Geometry check sheet. Reference: the model listing, model coordinates, mm. A direction names the side the tool comes from. Give positions to 0.01 mm unless a question says otherwise; leave off trailing zeros. Loops run counter-clockwise (first coordinate to the right, second up) from the corner with the lowest first, then second, coordinate; pieces in that order, holes last. Notation, with made-up numbers: (65, 75.5) -> (115, 75.5) arc R15 cw to (115, 79.5) -> close; hole circle Ø1 at (60.25, -26). An arc over 180 degrees is marked (long way). Write each question's results on one line, items separated by ' | '. Start each with the question number.
1) Draft check along X on faces 4 (the face through (67, 6, -75.8)), 5 (the face through (75.57, 6.08, -89.3)), 6 (the face through (56.019, 11.014, -79.626)), 7 (the face through (47, 10, -68)). Enter one of: pulls with the +X half, pulls with the -X half, needs draft (parallel to the pull), parting line crosses it, or undercut.
2) Sectioned sample at A-A on y = 1.5. Record the cut outline in (x, z), then the cut area to 3 significant figures.
3) Set-up check for faces 1 (the face through (62, 6, -61)), 2 (the face through (60, 5, -68)), 3 (the face through (37.92, 11.01, -78.84)): record each of +Z, -Z, +X, -X, +Y, -Y from which the full face is reachable in a straight line by a thin tool's end or side.
4) Depth check by flat-ended pin: pin 1 (13.5 mm diameter, centred on x = 43, z = -78.5, fed in from -Y); pin 2 (6 mm diameter, centred on y = 5.5, z = -60.5, fed in from +X); pin 3 (3 mm diameter, centred on x = 67, y = 8, fed in from +Z). Enter the tip coordinate at first touch or a pass-through.
5) Sectioned sample at C-C on z = -58.1. Record the cut outline in (x, y).
6) Scan lines: line 1 (X direction, y = 11.25, z = -58.1); line 2 (Z direction, x = 36.5, y = 11); line 3 (X direction, y = 3, z = -86). Record each from-to range of solid material in increasing order. Write a range as from..to.
7) Sectioned sample at B-B on x = 56.5. Record the cut outline in (y, z), then the cut area to 3 significant figures.
8) Sectioned sample at D-D on z = -81.5. Record the cut outline in (x, y).
```python
from build123d import *

# Parameters (mm, degrees)
SKETCH1_W           = 31
SKETCH1_H           = 45.4
BOSS_EXTRUDE1_DEPTH = 12
SKETCH2_W           = 27
SKETCH2_H           = 10
CUT_EXTRUDE1_DEPTH  = 57.268641356
SKETCH3_R           = 1.6
CUT_EXTRUDE2_DEPTH  = 10
SKETCH4_W           = 15
SKETCH4_H           = 12
BOSS_EXTRUDE2_DEPTH = 15
SKETCH5_R           = 1.6
CUT_EXTRUDE3_DEPTH  = 20
FILLET1_R           = 5


with BuildPart() as part:
    # Sketch1 → Boss-Extrude1 (new body)
    with BuildSketch(Plane(origin=(0, 0, 0), x_dir=(1, 0, 0), z_dir=(0, 1, 0))):
        with Locations((15.5, 22.7)):
            Rectangle(SKETCH1_W, SKETCH1_H)
    extrude(amount=BOSS_EXTRUDE1_DEPTH)

    # Sketch2 → Cut-Extrude1 (cut, through all)
    with BuildSketch(Plane.XY):
        with Locations((15.5, 5)):
            Rectangle(SKETCH2_W, SKETCH2_H)
    extrude(amount=-CUT_EXTRUDE1_DEPTH, mode=Mode.SUBTRACT)

    # Sketch3 → Cut-Extrude2 (cut)
    with BuildSketch(Plane(origin=(0, 12, 0), x_dir=(1, 0, 0), z_dir=(0, 1, 0))):
        with Locations(Location((5.5, 32.7, 0), (0, 0, 270))):
            Circle(SKETCH3_R)
        with Locations(Location((25.5, 32.7, 0), (0, 0, 270))):
            Circle(SKETCH3_R)
        with Locations(Location((25.5, 12.7, 0), (0, 0, 270))):
            Circle(SKETCH3_R)
        with Locations(Location((5.5, 12.7, 0), (0, 0, 270))):
            Circle(SKETCH3_R)
    extrude(amount=-CUT_EXTRUDE2_DEPTH, mode=Mode.SUBTRACT)

    # Sketch4 → Boss-Extrude2 (add)
    with BuildSketch(Plane.ZY):
        with Locations((-7.5, 6)):
            Rectangle(SKETCH4_W, SKETCH4_H)
    extrude(amount=BOSS_EXTRUDE2_DEPTH)

    # Sketch5 → Cut-Extrude3 (cut)
    with BuildSketch(Plane(origin=(0, 12, 0), x_dir=(1, 0, 0), z_dir=(0, 1, 0))):
        with Locations(Location((-10, 5, 0), (0, 0, 270))):
            Circle(SKETCH5_R)
    extrude(amount=-CUT_EXTRUDE3_DEPTH, mode=Mode.SUBTRACT)

    # Fillet1
    fillet1_edges = [part.edges().sort_by_distance(p)[0] for p in [
        (-15, 6, -15),
        (-15, 6, 0),
    ]]
    fillet(fillet1_edges, radius=FILLET1_R)


with BuildPart() as body_2:
    # Mirror2: mirrored copy
    add(part.part.mirror(Plane(origin=(31, 12, 0), x_dir=(0, 0, 1), z_dir=(-1, 0, 0))))


with BuildPart() as body_3:
    # Mirror3: mirrored copy
    add(body_2.part.mirror(Plane(origin=(62, 12, -45.4), x_dir=(1, 0, 0), z_dir=(0, 0, 1))))


solid = body_3.part
```
Result:
1) face 4: needs draft | face 5: pulls with the +X half | face 6: undercut | face 7: undercut
2) outline: (31, -90.8) -> (33, -90.8) -> (33, -45.4) -> (31, -45.4) -> close; (60, -90.8) -> (72, -90.8) arc R5 ccw to (77, -85.8) -> (77, -80.8) arc R5 ccw to (72, -75.8) -> (62, -75.8) -> (62, -45.4) -> (60, -45.4) -> close; hole circle Ø3.2 at (72, -85.8) | area: 388 mm^2
3) face 1: +Z, +X, +Y, -Y | face 2: +Z, -Z, -Y | face 3: +Y, -Y
4) pin 1: y = 10 | pin 2: x = 62 | pin 3: z = -75.8
5) outline: (31, 0) -> (33, 0) -> (33, 10) -> (34.9, 10) -> (34.9, 12) -> (31, 12) -> close; (38.1, 10) -> (54.9, 10) -> (54.9, 12) -> (38.1, 12) -> close; (58.1, 10) -> (60, 10) -> (60, 0) -> (62, 0) -> (62, 12) -> (58.1, 12) -> close
6) line 1: 31..34.9, 38.1..54.9, 58.1..62 | line 2: -90.8..-79.7, -76.5..-59.7, -56.5..-45.4 | line 3: 31..33, 60..70.41, 73.59..77
7) outline: (10, -90.8) -> (12, -90.8) -> (12, -79.7) -> (10, -79.7) -> close; (10, -76.5) -> (12, -76.5) -> (12, -59.7) -> (10, -59.7) -> close; (10, -56.5) -> (12, -56.5) -> (12, -45.4) -> (10, -45.4) -> close | area: 78.0 mm^2
8) outline: (31, 0) -> (33, 0) -> (33, 10) -> (60, 10) -> (60, 0) -> (77, 0) -> (77, 12) -> (31, 12) -> close
